Part model, mm, in its own coordinate system. Face numbers are marked on the shaded views. A direction names the side the tool comes from. Round coordinates to 2 decimals unless told otherwise and drop trailing zeros. Loops run counter-clockwise (first coordinate to the right, second up) from the corner with the lowest first, then second, coordinate; pieces in that order, holes last. Notation, with made-up numbers: M 69.5,50.5 L 87.5,50.5 A34 cw 87.5,88.5 Z; hole C -34.5,18.25 d10. An arc over 180 degrees is marked long. Write each question's results on one line, items separated by ' | '.
from build123d import *

# Parameters (mm, degrees)
SKETCH1_R           = 8.2
BOSS_EXTRUDE1_DEPTH = 10
SKETCH2_R           = 1.585
CUT_EXTRUDE1_DEPTH  = 10


with BuildPart() as part:
    # Sketch1 → Boss-Extrude1 (new body)
    with BuildSketch(Plane.XY):
        with BuildLine():
            Line((-4.18853286, 12.607697881), (-4.18853286, 5.367776119))
            Line((-4.18853286, 5.367776119), (-10.519480519, 5.367776119))
            Line((-10.519480519, 5.367776119), (-10.519480519, 0.367776119))
            Line((-10.519480519, 0.367776119), (39.480519481, 0.367776119))
            Line((39.480519481, 0.367776119), (39.480519481, 5.367776119))
            Line((39.480519481, 5.367776119), (31.405454323, 5.367776119))
            Line((31.405454323, 5.367776119), (31.410877884, 12.433894833))
            ThreePointArc((31.410877884, 12.433894833), (26.812708154, 29.608501659), (22.010917954, 12.489708029))
            Line((22.010917954, 12.489708029), (22.005451554, 5.367776119))
            Line((22.005451554, 5.367776119), (5.205765597, 5.367776119))
            Line((5.205765597, 5.367776119), (5.205765597, 12.316995042))
            ThreePointArc((5.205765597, 12.316995042), (1.04612148, 29.83226088), (-4.18853286, 12.607697881))
        make_face()
        with Locations((26.753246753, 20.367776119)):
            Circle(SKETCH1_R, mode=Mode.SUBTRACT)
        with Locations((0.753246753, 20.367776119)):
            Circle(SKETCH1_R, mode=Mode.SUBTRACT)
    extrude(amount=BOSS_EXTRUDE1_DEPTH)

    # Sketch2 → Cut-Extrude1 (cut)
    with BuildSketch(Plane(origin=(0, 5.367776119, 0), x_dir=(1, 0, 0), z_dir=(0, 1, 0))):
        with Locations(Location((13.958626021, -5.067111952, 0), (0, 0, 270))):
            Circle(SKETCH2_R)
    extrude(amount=-CUT_EXTRUDE1_DEPTH, mode=Mode.SUBTRACT)


solid = part.part
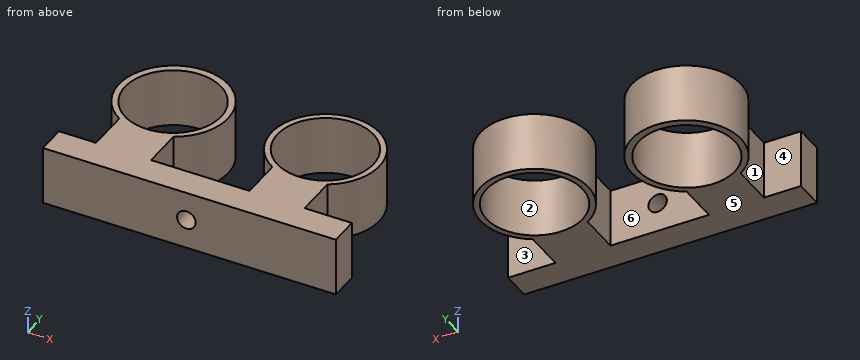
Item 1: Band-saw the part on D-D on x = 6. Give the cut face in (y, z), and give its area (3 significant figures).
Filled sheet:
outline: M 0.37,0 L 5.37,0 L 5.37,10 L 0.37,10 Z; M 12.8,0 L 14.07,0 L 14.07,10 L 12.8,10 Z; M 26.67,0 L 28.22,0 L 28.22,10 L 26.67,10 Z | area: 78.2 mm^2
Item 2: Band-saw the part on B-B on x = 27.5. Give the cut face in (y, z), and give its area (3 significant figures).
Filled sheet:
outline: M 0.37,0 L 12.2,0 L 12.2,10 L 0.37,10 Z; M 28.53,0 L 29.58,0 L 29.58,10 L 28.53,10 Z | area: 129 mm^2
Item 3: Band-saw the part on A-A on z = 5.5. Give the cut face in (x, y), and give its area (3 significant figures).
Filled sheet:
outline: M -10.52,0.37 L 12.43,0.37 L 12.43,5.37 L 5.21,5.37 L 5.21,12.32 A9.32 ccw long -4.19,12.61 L -4.19,5.37 L -10.52,5.37 Z; M 15.48,0.37 L 39.48,0.37 L 39.48,5.37 L 31.41,5.37 L 31.41,12.43 A9.22 ccw long 22.01,12.49 L 22.01,5.37 L 15.48,5.37 Z; hole C 0.75,20.37 d16.4; hole C 26.75,20.37 d16.4 | area: 469 mm^2
Item 4: Wall check: L1, parallel to X at y = 19.75, z = 6; L2, parallel to X at y = 13.5, z = 5.75; L3, parallel to Y at x = 20, z = 6.75. Give the ranges that are in metal, low to high.
Filled sheet:
L1: -8.54 to -7.42, 8.93 to 10.05, 17.56 to 18.58, 34.93 to 35.95 | L2: -5.39 to -3.73, 5.23 to 6.9, 20.64 to 22.27, 31.23 to 32.88 | L3: 0.37 to 5.37, 14.12 to 15.72, 25.02 to 26.66
Item 5: Which spindle directions (+Z, -Z, +X, -X, +Y, -Y) get a long thin tool onto all of the face, cutting with end or side? Do the marked faces 4, 5 and 6. Say none if no direction does.
Filled sheet:
face 4: +Z, -Z, -X | face 5: -Z, +X, -X, +Y, -Y | face 6: +Z, -Z
Item 6: Two-plate mould, pull along X, no slides. Class the marked faces 1, 2 and 3: +X half, -X half, draft (parallel to the pull), parting line (faces both ways), or undercut.
Filled sheet:
face 1: -X half | face 2: undercut | face 3: draft
Item 7: Band-saw the part on C-C on y = 24.75. Give the cut face in (x, z), and give its area (3 significant figures).
Filled sheet:
outline: M -7.55,0 L -6.18,0 L -6.18,10 L -7.55,10 Z; M 7.68,0 L 9.06,0 L 9.06,10 L 7.68,10 Z; M 18.64,0 L 19.82,0 L 19.82,10 L 18.64,10 Z; M 33.68,0 L 34.88,0 L 34.88,10 L 33.68,10 Z | area: 51.3 mm^2
Item 8: Drop flat-ended pins along their axis: P1, Ø3, axis at y = 17, z = 5, coming from the -X side; P2, Ø3.5, axis at y = 10, z = 3.5, coming from the +X side; P3, Ø3, axis at y = 15, z = 8, coming from the +X side. Give the stop position or say it passes through.
Filled sheet:
P1: x = -8.35 | P2: x = 31.41 | P3: x = 35.11
